from build123d import *

# Parameters (mm, degrees)
SKETCH1_R           = 1
SKETCH1_R_2         = 1.3
BOSS_EXTRUDE1_DEPTH = 1.6


with BuildPart() as part:
    # Sketch1 → Boss-Extrude1 (new body)
    with BuildSketch(Plane(origin=(0, 0, 0), x_dir=(1, 0, 0), z_dir=(0, 1, 0))):
        Polygon((0, 0), (61, 0), (61, 2), (65, 2), (65, 0), (70, 0), (70, 12.7), (65, 12.7), (65, 10.7), (61, 10.7), (61, 12.7), (0, 12.7), align=None)
        with Locations(Location((4, 9.525, 0), (0, 0, 270))):
            Circle(SKETCH1_R, mode=Mode.SUBTRACT)
        with Locations(Location((4, 3.175, 0), (0, 0, 270))):
            Circle(SKETCH1_R, mode=Mode.SUBTRACT)
        with Locations(Location((25, 6.35, 0), (0, 0, 270))):
            Circle(SKETCH1_R_2, mode=Mode.SUBTRACT)
        with Locations(Location((45, 6.35, 0), (0, 0, 90))):
            Circle(SKETCH1_R_2, mode=Mode.SUBTRACT)
    extrude(amount=BOSS_EXTRUDE1_DEPTH)


solid = part.part
Geometry check sheet. Reference: the model listing, model coordinates, mm. A direction names the side the tool comes from. Round coordinates to 2 decimals unless told otherwise and drop trailing zeros. Order: outer loops, then holes, each group sorted by start corner. A loop starts at its lowest first (then second) coordinate and runs counter-clockwise, first axis right, second up. Notation, with made-up numbers: M 70,59 L 98,59 A9 ccw 98,64 Z; hole C 20,17.25 d5. An arc over 180 degrees is marked long. Answer in a Markdown table with one row per item.
(1) Sectioned sample at B-B, the plane z = -6.35. Record the cut outline in (x, y), and give its area (3 significant figures).
Responses:
| item | result |
|---|---|
| outline | M 0,0 L 23.7,0 L 23.7,1.6 L 0,1.6 Z; M 26.3,0 L 43.7,0 L 43.7,1.6 L 26.3,1.6 Z; M 46.3,0 L 70,0 L 70,1.6 L 46.3,1.6 Z |
| area | 104 mm² |
(2) Draft check along Z on faces 1 (the face through (4.68, 0.79, -3.91)), 2 (the face through (35, 0, -6)), 3 (the face through (31, 1, -12.7)), 4 (the face through (23.73, 0.79, -6.63)). Enter one of: released by +Z, released by -Z, zero draft, split by the parting line, or undercut.
Responses:
| item | result |
|---|---|
| face 1 | undercut |
| face 2 | zero draft |
| face 3 | released by -Z |
| face 4 | undercut |
(3) Go/stop test with a flat-tipped pin: P1, Ø0.8, axis at x = 63, y = 0.5, coming from the +Z side. Record where the tip stops, or that it passes through.
Responses:
| item | result |
|---|---|
| P1 | stops at z = -2 |
(4) Sectioned sample at C-C, the plane y = 0.35. Record the cut outline in (x, z) (3 decimals).
Responses:
| item | result |
|---|---|
| outline | M 0,-12.7 L 61,-12.7 L 61,-10.7 L 65,-10.7 L 65,-12.7 L 70,-12.7 L 70,0 L 65,0 L 65,-2 L 61,-2 L 61,0 L 0,0 Z; hole C 4,-9.525 d2; hole C 4,-3.175 d2; hole C 25,-6.35 d2.6; hole C 45,-6.35 d2.6 |
(5) Sectioned sample at D-D, the plane x = 4. Record the cut outline in (y, z) (3 decimals), and give its area (3 significant figures).
Responses:
| item | result |
|---|---|
| outline | M 0,-12.7 L 1.6,-12.7 L 1.6,-10.525 L 0,-10.525 Z; M 0,-8.525 L 1.6,-8.525 L 1.6,-4.175 L 0,-4.175 Z; M 0,-2.175 L 1.6,-2.175 L 1.6,0 L 0,0 Z |
| area | 13.9 mm² |
(6) Tool access check on faces 5 (the face through (67, 1, 0)), 6 (the face through (65, 1, -12)), 7 (the face through (63, 1, -2)). Record the directions out of +Z, -Z, +X, -X, +Y, -Y that give a thin tool (end or side, any length) a straight path to the whole face; none if there is none.
Responses:
| item | result |
|---|---|
| face 5 | +Z, +X, -X, +Y, -Y |
| face 6 | -Z, +Y, -Y |
| face 7 | +Z, +Y, -Y |
(7) Sectioned sample at A-A, the plane x = 25. Record the cut outline in (y, z).
Responses:
| item | result |
|---|---|
| outline | M 0,-12.7 L 1.6,-12.7 L 1.6,-7.65 L 0,-7.65 Z; M 0,-5.05 L 1.6,-5.05 L 1.6,0 L 0,0 Z |
(8) Scan lines: probe 1 along X at (y, z) = (0.55, -6.35); probe 2 along Z at (x, y) = (45, 1.1); probe 3 along X at (y, z) = (1, -1). Record each from-to range of solid material in increasing order. Write a range as from..to.
Responses:
| item | result |
|---|---|
| probe 1 | x = 0..23.7, 26.3..43.7, 46.3..70 |
| probe 2 | z = -12.7..-7.65, -5.05..0 |
| probe 3 | x = 0..61, 65..70 |
